The figure shows three views and two pictorial views of one solid part (mm, origin at its lowest corner). Answer the questions. Coordinates: 2 decimals unless noted, no trailing zeros. Order: outer loops, then holes, each group sorted by start corner. A loop starts at its lowest first (then second) coordinate and runs counter-clockwise, first axis right, second up. Notation, with made-up numbers: M 44,65.25 L 84,65.25 A9 ccw 84,81.25 Z; hole C 6,60.25 d2. An arc over 180 degrees is marked long. Write item = value, one per line. Start each with the question number.
Q1. This flat-tipped pin is pushed along its axis until it touches: P1, Ø4, axis at x = 15, y = 33.5, coming from the +Z side. Where does it stop, or does it pass through?
Q2. Find section B-B on y = 19. Give the vertices of the cut face in (x, z) (1 decimal).
Q3. Find section A-A on x = 2.5. Give the number of separate pieces and of enclosed holes in the cut face, and give its area (3 significant figures).
Q4. Straight lines are drawn through the part: line 1 along Y through (x, z) = (18.5, 5.5); line 2 along Z through (x, y) = (34.5, 39.05) (1 decimal); line 3 along Z through (x, y) = (2, 1) (1 decimal). For each, find the intervals that lie inside material, in ascending order.
Q5. Determine the mould class of the marked faces 1, 2, 3 and 4 for opening direction Y: released by +Y, released by -Y, zero draft, split by the parting line, or undercut.
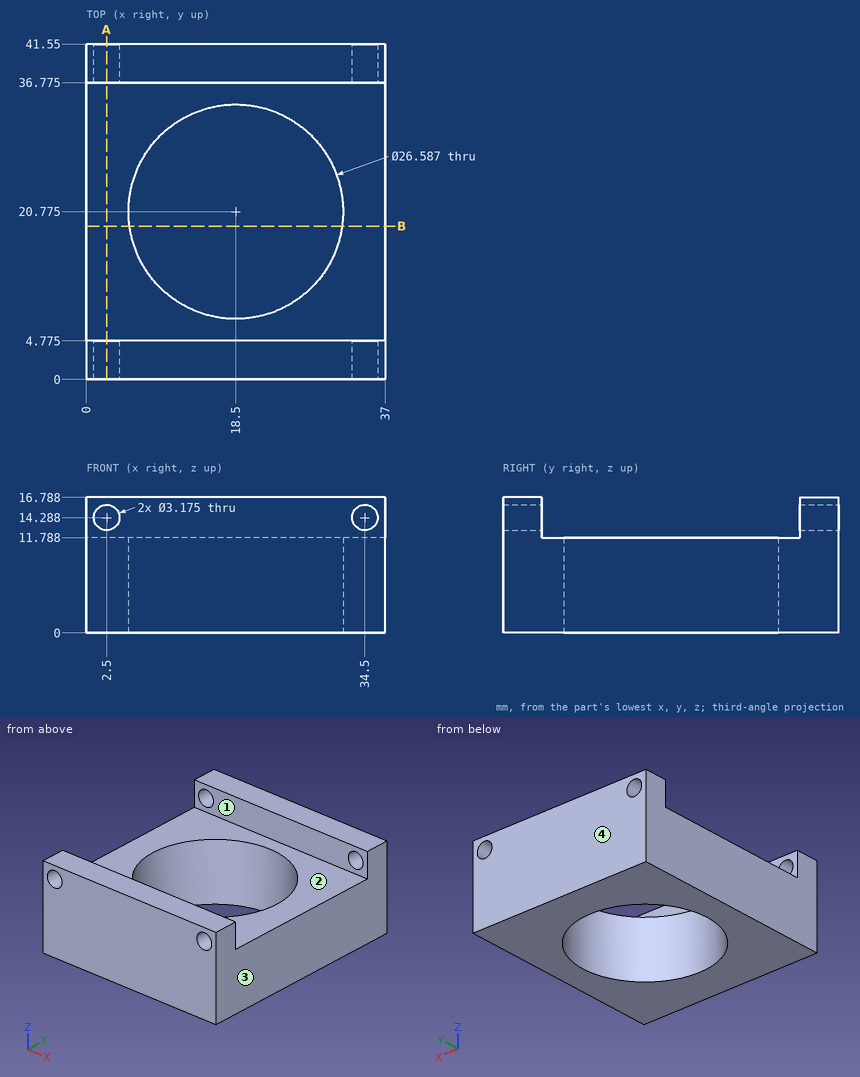
Findings below:
q1.P1 = 11.79
q2.outline = M 0,0 L 5.3,0 L 5.3,11.8 L 0,11.8 Z; M 31.7,0 L 37,0 L 37,11.8 L 31.7,11.8 Z
q3.separate_pieces = 3
q3.enclosed_holes = 0
q3.area = 507 mm^2
q4.line_1 = 0 to 7.48, 34.07 to 41.55
q4.line_2 = 0 to 12.7, 15.9 to 16.8
q4.line_3 = 0 to 12.8, 15.8 to 16.8
q5.face_1 = undercut
q5.face_2 = undercut
q5.face_3 = zero draft
q5.face_4 = released by +Y
